Source: three-view drawing plus pictorial views. Frame: mm from the lowest corner of the part. Give positions to 0.01 mm unless a question says otherwise; leave off trailing zeros. Write each loop counter-clockwise with the first axis right and the second up, starting at its lowest first coordinate (ties: lowest second). Pieces come first, ordered by that corner, then holes. Notation, with made-up numbers: (65.5, -26.5) -> (123.5, -26.5) arc R21 cw to (123.5, 2.5) -> close; hole circle Ø6 at (89.25, -30). An arc over 180 degrees is marked (long way). Answer in a Markdown table with one row per item. Add a question column.
Item 1: Section query C-C on x = 160.5. Output: boundary loops of the cut face in (y, z), plus the area to 3 significant figures.
Item 2: First-contact query: P1, Ø1.6, axis at x = 22.5, z = 1, coming from the +Y side; P2, Ø1.5, axis at y = 1, z = 2, coming from the -X side; P3, Ø0.9, axis at y = 2, z = 2, coming from the +X side. Flat tips, straight axial feed; report the tip coordinate or a pass-through.
Item 3: Section query B-B on z = 1.3. Output: boundary loops of the cut face in (x, y).
Item 4: Material intervals for probe 1 along Y at (x, z) = (104.5, 1.4); probe 2 along X at (y, z) = (61, 2); probe 3 along Y at (x, z) = (13.5, 2.25), sorted ascending. Write a range as from..to.
Item 5: Section query A-A on y = 64.5. Output: boundary loops of the cut face in (x, z).
Item 6: Section query D-D on x = 18. Output: boundary loops of the cut face in (y, z).
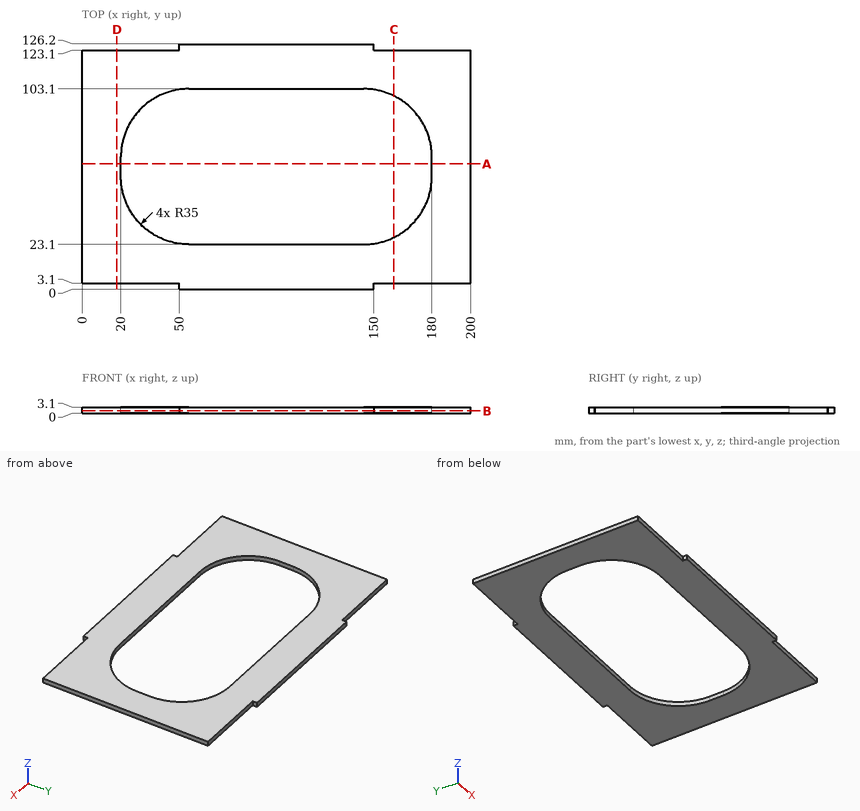
Findings below:
| question | item | result |
|---|---|---|
| 1 | outline | (3.1, 0) -> (26.72, 0) -> (26.72, 3.1) -> (3.1, 3.1) -> close; (99.48, 0) -> (123.1, 0) -> (123.1, 3.1) -> (99.48, 3.1) -> close |
| 1 | area | 146 mm^2 |
| 2 | P1 | stops at y = 123.1 |
| 2 | P2 | stops at x = 50 |
| 2 | P3 | stops at x = 150 |
| 3 | outline | (0, 3.1) -> (50, 3.1) -> (50, 0) -> (150, 0) -> (150, 3.1) -> (200, 3.1) -> (200, 123.1) -> (150, 123.1) -> (150, 126.2) -> (50, 126.2) -> (50, 123.1) -> (0, 123.1) -> close; hole (20, 58.1) arc R35 ccw to (55, 23.1) -> (145, 23.1) arc R35 ccw to (180, 58.1) -> (180, 68.1) arc R35 ccw to (145, 103.1) -> (55, 103.1) arc R35 ccw to (20, 68.1) -> close |
| 4 | probe 1 | y = 0..23.1, 103.1..126.2 |
| 4 | probe 2 | x = 0..20, 180..200 |
| 4 | probe 3 | y = 3.1..123.1 |
| 5 | outline | (0, 0) -> (20, 0) -> (20, 3.1) -> (0, 3.1) -> close; (180, 0) -> (200, 0) -> (200, 3.1) -> (180, 3.1) -> close |
| 6 | outline | (3.1, 0) -> (123.1, 0) -> (123.1, 3.1) -> (3.1, 3.1) -> close |
